Input: part model. Units: mm. Frame: model coordinates. Give positions to 0.01 mm unless a question says otherwise; leave off trailing zeros. Loops run counter-clockwise (first coordinate to the right, second up) from the corner with the lowest first, then second, coordinate; pieces in that order, holes last. Notation, with made-up numbers: (81.5, -30.5) -> (121.5, -30.5) arc R25 ccw to (121.5, -7.5) -> close; hole circle Ø9 at (68, 76.5). An arc over 180 degrees is marked (long way). Answer as a JSON object with one key per item and string values.
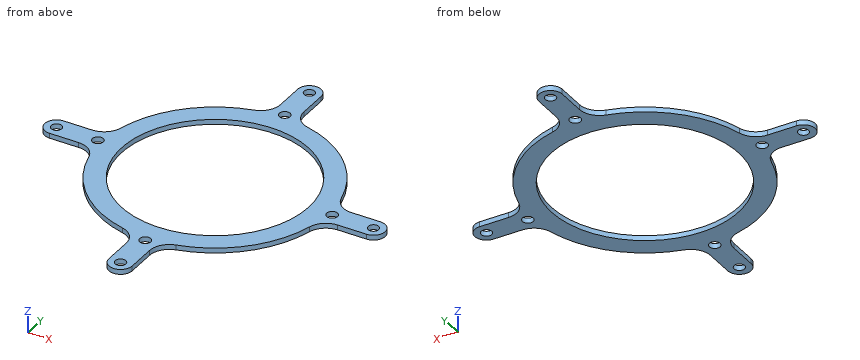
```python
from build123d import *

# Parameters (mm, degrees)
SKETCH_1_R          = 34.15
SKETCH_1_R_2        = 28.15
SKETCH_1_R_3        = 1.6
EXTRUDE_1_DEPTH     = 1.5
FILLET_1_R          = 6
SKETCH_3_R          = 1.65
CUT_EXTRUDE_1_DEPTH = 3


with BuildPart() as part:
    # 草图1 → 凸台-拉伸1 (new body)
    # profile 1 of 5: a face of its own
    with BuildSketch(Plane.XY):
        Circle(SKETCH_1_R)
        Circle(SKETCH_1_R_2, mode=Mode.SUBTRACT)
    # profile 2 of 5: a face of its own
    with BuildSketch(Plane.XY):
        with BuildLine():
            Line((3.5, 47.7), (3.5, 34.15))
            ThreePointArc((3.5, 34.15), (0, 30.65), (-3.5, 34.15))
            Line((-3.5, 34.15), (-3.5, 47.7))
            ThreePointArc((-3.5, 47.7), (0, 51.2), (3.5, 47.7))
        make_face()
        with Locations((0, 47.7)):
            Circle(SKETCH_1_R_3, mode=Mode.SUBTRACT)
    # profile 3 of 5: a face of its own
    with BuildSketch(Plane.XY):
        with BuildLine():
            Line((47.7, -3.5), (34.15, -3.5))
            ThreePointArc((34.15, -3.5), (30.65, 0), (34.15, 3.5))
            Line((34.15, 3.5), (47.7, 3.5))
            ThreePointArc((47.7, 3.5), (51.2, 0), (47.7, -3.5))
        make_face()
        with Locations((47.7, 0)):
            Circle(SKETCH_1_R_3, mode=Mode.SUBTRACT)
    # profile 4 of 5: a face of its own
    with BuildSketch(Plane.XY):
        with BuildLine():
            Line((-3.5, -47.7), (-3.5, -34.15))
            ThreePointArc((-3.5, -34.15), (0, -30.65), (3.5, -34.15))
            Line((3.5, -34.15), (3.5, -47.7))
            ThreePointArc((3.5, -47.7), (0, -51.2), (-3.5, -47.7))
        make_face()
        with Locations((0, -47.7)):
            Circle(SKETCH_1_R_3, mode=Mode.SUBTRACT)
    # profile 5 of 5: a face of its own
    with BuildSketch(Plane.XY):
        with BuildLine():
            Line((-47.7, 3.5), (-34.15, 3.5))
            ThreePointArc((-34.15, 3.5), (-30.65, 0), (-34.15, -3.5))
            Line((-34.15, -3.5), (-47.7, -3.5))
            ThreePointArc((-47.7, -3.5), (-51.2, 0), (-47.7, 3.5))
        make_face()
        with Locations((-47.7, 0)):
            Circle(SKETCH_1_R_3, mode=Mode.SUBTRACT)
    extrude(amount=EXTRUDE_1_DEPTH)

    # 圆角1
    fillet_1_edges = [part.edges().sort_by_distance(p)[0] for p in [
        (-3.49540148, 33.970644217, 0.75),
        (3.49540148, 33.970644217, 0.75),
        (33.970644217, 3.49540148, 0.75),
        (33.970644217, -3.49540148, 0.75),
        (3.49540148, -33.970644217, 0.75),
        (-3.49540148, -33.970644217, 0.75),
        (-33.970644217, -3.49540148, 0.75),
        (-33.970644217, 3.49540148, 0.75),
    ]]
    fillet(fillet_1_edges, radius=FILLET_1_R)

    # 草图3 → 切除-拉伸1 (cut)
    with BuildSketch(Plane.XY.offset(1.5)):
        with Locations((-35.25, 0)):
            Circle(SKETCH_3_R)
        with Locations((0, 35.25)):
            Circle(SKETCH_3_R)
        with Locations((35.25, 0)):
            Circle(SKETCH_3_R)
        with Locations((0, -35.25)):
            Circle(SKETCH_3_R)
    extrude(amount=-CUT_EXTRUDE_1_DEPTH, mode=Mode.SUBTRACT)


solid = part.part
```
Q1. Pin query (flat end, axial travel): pin 1 (0.5 mm diameter, centred on y = 42.5, z = 0.5, fed in from -X); pin 2 (4 mm diameter, centred on x = 0, y = -35.25, fed in from +Z); pin 3 (0.8 mm diameter, centred on y = -43, z = 0.5, fed in from +X); pin 4 (0.8 mm diameter, centred on x = -42, z = 0.5, fed in from -Y). Return the tip coordinate at first contact, or that it passes through.
Evaluation:
{"pin 1": "stops at x = -3.5", "pin 2": "stops at z = 1.5", "pin 3": "stops at x = 3.5", "pin 4": "stops at y = -3.5"}
Q2. Section A-A, the plane x = 0. Return the cut outline in (y, z), then the cut area to 4 significant figures.
Evaluation:
{"outline": "(-51.2, 0) -> (-49.3, 0) -> (-49.3, 1.5) -> (-51.2, 1.5) -> close; (-46.1, 0) -> (-36.9, 0) -> (-36.9, 1.5) -> (-46.1, 1.5) -> close; (-33.6, 0) -> (-28.15, 0) -> (-28.15, 1.5) -> (-33.6, 1.5) -> close; (28.15, 0) -> (33.6, 0) -> (33.6, 1.5) -> (28.15, 1.5) -> close; (36.9, 0) -> (46.1, 0) -> (46.1, 1.5) -> (36.9, 1.5) -> close; (49.3, 0) -> (51.2, 0) -> (51.2, 1.5) -> (49.3, 1.5) -> close", "area": "49.65 mm2"}
Q3. Section D-D, the plane y = -19.5. Return the cut outline in (x, z), then the cut area to 3 significant figures.
Evaluation:
{"outline": "(-28.04, 0) -> (-20.3, 0) -> (-20.3, 1.5) -> (-28.04, 1.5) -> close; (20.3, 0) -> (28.04, 0) -> (28.04, 1.5) -> (20.3, 1.5) -> close", "area": "23.2 mm2"}
Q4. Ray query, line 1 along Y through (x, z) = (0, 0.3); line 2 along Y through (x, z) = (1, 1); line 3 along Y through (x, z) = (47.7, 0.9). Return the intervals inside material, ascending.
Evaluation:
{"line 1": "y = -51.2 to -49.3, -46.1 to -36.9, -33.6 to -28.15, 28.15 to 33.6, 36.9 to 46.1, 49.3 to 51.2", "line 2": "y = -51.05 to -48.95, -46.45 to -36.56, -33.94 to -28.13, 28.13 to 33.94, 36.56 to 46.45, 48.95 to 51.05", "line 3": "y = -3.5 to -1.6, 1.6 to 3.5"}
Q5. Section C-C, the plane x = 13. Return the cut outline in (y, z), then the cut area to 3 significant figures.
Evaluation:
{"outline": "(-31.58, 0) -> (-24.97, 0) -> (-24.97, 1.5) -> (-31.58, 1.5) -> close; (24.97, 0) -> (31.58, 0) -> (31.58, 1.5) -> (24.97, 1.5) -> close", "area": "19.8 mm2"}
